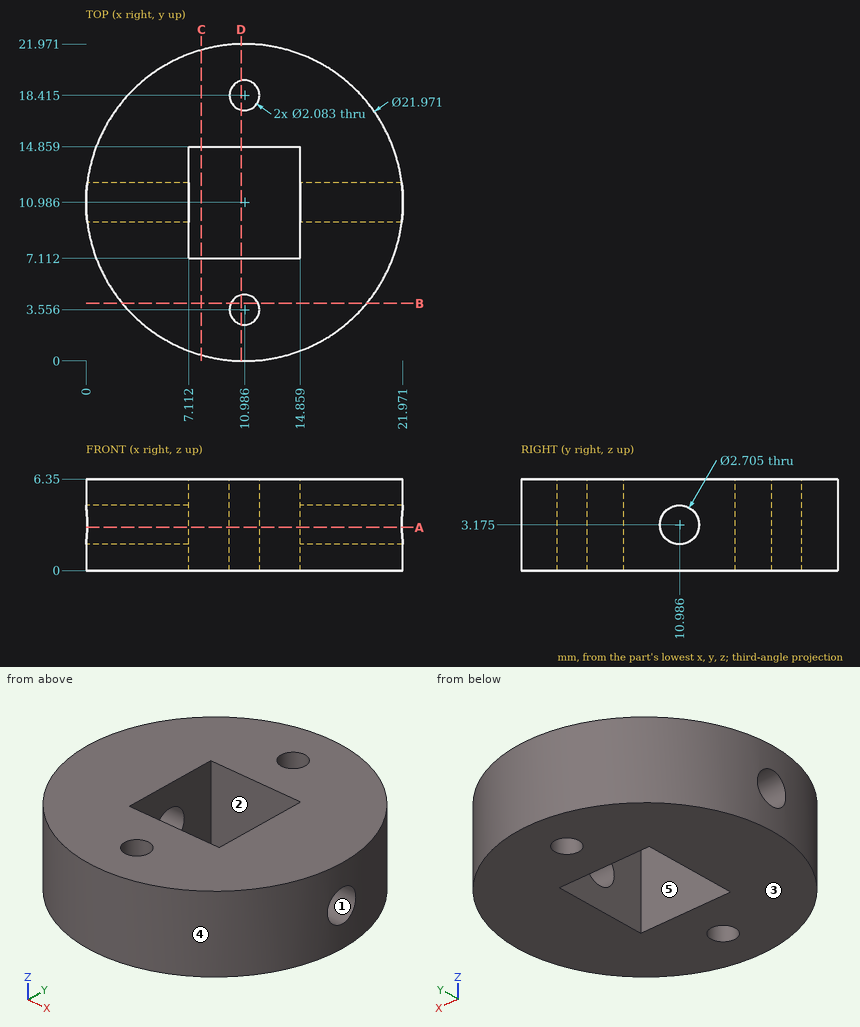
For this review, use the dimensioned drawing (mm, ordinates from the lowest corner) and the shaded views. A direction names the side the tool comes from. Give positions to 0.01 mm unless a question says otherwise; leave off trailing zeros. Write each loop counter-clockwise with the first axis right and the second up, starting at its lowest first coordinate (ties: lowest second). Pieces come first, ordered by that corner, then holes.
(1) Consider section B-B, the plane y = 4. Give the boundary of the cut face in (x, z).
(2) Tool access review of the marked faces 1 and 2: name each direction out of +Z, -Z, +X, -X, +Y, -Y from which nothing blocks a thin tool from reaching the whole face with its end or side.
(3) To check wall thickness, follow L1, parallel to Y at x = 11.25, z = 4; L2, parallel to X at y = 14, z = 1.5; L3, parallel to X at y = 12.75, z = 3.75. State the ranges of each line that lie inside material, in increasing order.
(4) Consider section A-A, the plane z = 3. Give the boundary of the cut face in (x, y) (1 decimal), and give its area (3 significant figures).
(5) The part is to be moulded in two halves that separate along Y. For the marked faces 3, 4 and 5, say which applies: released by +Y, released by -Y, zero draft, split by the parting line, or undercut.
(6) Consider section D-D, the plane x = 10.75. Give the boundary of the cut face in (y, z).
(7) Consider section C-C, the plane x = 8. Give the boundary of the cut face in (y, z).
(8) For P1, Ø3, axis at y = 16, z = 1, coming from the -X side; P2, Ø1.9, axis at x = 9.5, z = 2, coming from the +Y side; P3, Ø1.9, axis at y = 12.5, z = 3.5, coming from the +X side, all flat-tipped, find the tip position at first contact; note any pin that passes through.
Returned:
1. outline: (2.51, 0) - (10.04, 0) - (10.04, 6.35) - (2.51, 6.35) - close; (11.93, 0) - (19.46, 0) - (19.46, 6.35) - (11.93, 6.35) - close
2. face 1: +X, -X
2. face 2: +Z, -Z
3. L1: y = 0 to 2.55, 4.56 to 7.11, 14.86 to 17.41, 19.42 to 21.97
3. L2: x = 0.42 to 7.11, 14.86 to 21.55
3. L3: x = 0.14 to 7.11, 14.86 to 21.83
4. outline: (0.1, 9.6) arc R11 ccw to (21.9, 9.6) - (14.9, 9.6) - (14.9, 7.1) - (7.1, 7.1) - (7.1, 9.6) - close; (0.1, 12.3) - (7.1, 12.3) - (7.1, 14.9) - (14.9, 14.9) - (14.9, 12.3) - (21.9, 12.3) arc R11 ccw to start; hole circle Ø2.1 at (11, 3.6); hole circle Ø2.1 at (11, 18.4)
4. area: 274 mm2
5. face 3: zero draft
5. face 4: split by the parting line
5. face 5: undercut
6. outline: (0, 0) - (2.54, 0) - (2.54, 6.35) - (0, 6.35) - close; (4.57, 0) - (7.11, 0) - (7.11, 6.35) - (4.57, 6.35) - close; (14.86, 0) - (17.4, 0) - (17.4, 6.35) - (14.86, 6.35) - close; (19.43, 0) - (21.97, 0) - (21.97, 6.35) - (19.43, 6.35) - close
7. outline: (0.41, 0) - (7.11, 0) - (7.11, 6.35) - (0.41, 6.35) - close; (14.86, 0) - (21.56, 0) - (21.56, 6.35) - (14.86, 6.35) - close
8. P1: stops at x = 0.58
8. P2: stops at y = 21.96
8. P3: stops at x = 21.94
